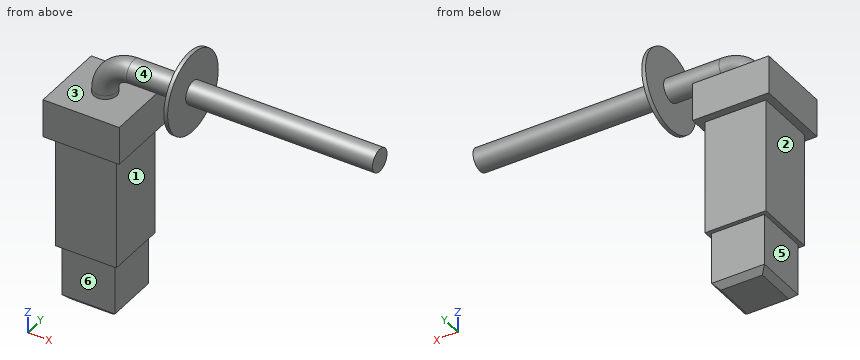
from build123d import *

# Parameters (mm, degrees)
F0_W      = 27.8
F0_H      = 27.8
F1_DEPTH  = 30
F2_W      = 32
F2_H      = 32
F2_W_2    = 27.8
F2_H_2    = 27.8
F3_DEPTH  = 80
F4_W      = 40
F4_H      = 40
F5_DEPTH  = 20
F7_R      = 6
F10_R     = 21
F11_DEPTH = 2
F12_SIZE  = 3


with BuildPart() as f1:
    # F0 (on Top) → F1 (new body)
    with BuildSketch(Plane.XY):
        Rectangle(F0_W, F0_H)
    extrude(amount=F1_DEPTH)

    # F2 (on face) → F3 (join)
    with BuildSketch(Plane.XY.offset(30)):
        Rectangle(F2_W, F2_H)
        Rectangle(F2_W_2, F2_H_2, mode=Mode.SUBTRACT)
        Rectangle(F2_W_2, F2_H_2)
    extrude(amount=F3_DEPTH)

    # F4 (on face) → F5 (join)
    with BuildSketch(Plane.XY.offset(110)):
        Rectangle(F4_W, F4_H)
    extrude(amount=-F5_DEPTH)

    # F8: sweep along a path in F6
    with BuildLine(Plane.XZ) as f8_path:
        Line((0, 110), (0, 112))
        ThreePointArc((0, 112), (4.3933982822, 122.6066017178), (15, 127))
        Line((15, 127), (144, 127))
    # F7 (on face) → F8 (sweep)
    with BuildSketch(Plane.XY.offset(110)):
        Circle(F7_R)
    sweep(path=f8_path.line)

    # F10 (on offset) → F11 (join)
    with BuildSketch(Plane.YZ.offset(44)):
        with Locations((0, 127)):
            Circle(F10_R)
    extrude(amount=F11_DEPTH)

    # F12
    f12_edges = [f1.edges().sort_by_distance(p)[0] for p in [
        (0, -13.9, 0),
        (13.9, 0, 0),
        (0, 13.9, 0),
        (-13.9, 0, 0),
    ]]
    chamfer(f12_edges, length=F12_SIZE)


solid = f1.part
Here's how the part is built. I have some questions about the finished solid (model axes, mm). Face numbers are marked on the shaded views. A direction names the side the tool comes from. Coordinates: 2 decimals unless noted, no trailing zeros. Loops run counter-clockwise (first coordinate to the right, second up) from the corner with the lowest first, then second, coordinate; pieces in that order, holes last. Notation, with made-up numbers: (49.25, -30) -> (100.25, -30) arc R4 cw to (100.25, -26) -> close; hole circle Ø10 at (33.25, -7). An arc over 180 degrees is marked (long way). Use one line per item in the form item = value. Start each with the question number.
(1) We'd pull the mould along X, two halves only. Please class the marked faces 4, 5 and 6: pulls with the +X half, pulls with the -X half, needs draft (parallel to the pull), parting line crosses it, or undercut.
(2) If we section it at C-C (z = 88): Please give me the cut outline in (x, y), then the cut area to 3 significant figures.
(3) Please list where these lines run through material, in increasing order: line 1 along X through (y, z) = (-10, 103.5); line 2 along X through (y, z) = (-4, 8.5).
(4) If we section it at B-B (x = 107.5): Please give me the cut outline in (y, z), then the cut area to 3 significant figures.
(5) On a 3-axis mill with a long thin cutter (end or side, diameter ignored), from which of +Z, -Z, +X, -X, +Y, -Y can I reach the whole of each face in a straight line? I mean the marked faces 1, 2 and 3. Say none if no direction works.
(6) Will these pins go through, and if not, where does the flat tip stop? pin 1 (8 mm diameter, centred on x = 3, z = 19, fed in from +Y); pin 2 (21.5 mm diameter, centred on y = 2, z = 12, fed in from +X); pin 3 (10 mm diameter, centred on y = 8, z = 97.5, fed in from +X).
Verdict:
q1.face_4 = undercut
q1.face_5 = pulls with the -X half
q1.face_6 = needs draft
q2.outline = (-16, -16) -> (16, -16) -> (16, 16) -> (-16, 16) -> close
q2.area = 1,020 mm²
q3.line_1 = -20 to 20
q3.line_2 = -13.9 to 13.9
q4.outline = circle Ø12 at (0, 127)
q4.area = 113 mm²
q5.face_1 = -Z, +X, +Y, -Y
q5.face_2 = -Z, -X, +Y, -Y
q5.face_3 = none
q6.pin_1 = 13.9
q6.pin_2 = 13.9
q6.pin_3 = 20
